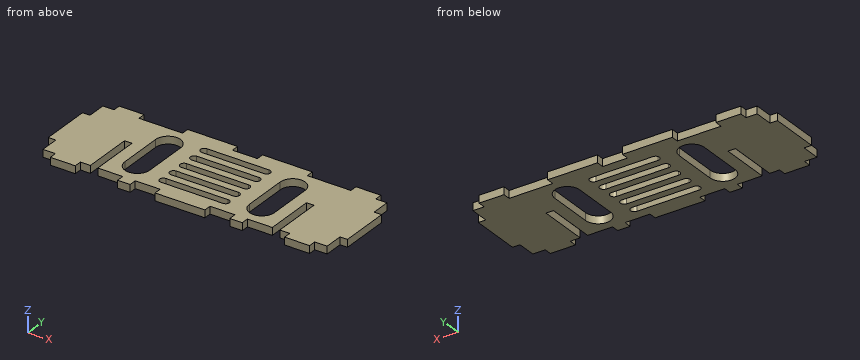
Autodesk Inventor part; units mm, degrees
ref_plane "YZ Plane" through (0, 0, 0) normal (1, 0, 0) x (0, 1, 0)
ref_plane "XZ Plane" through (0, 0, 0) normal (0, 1, 0) x (-1, 0, 0)
ref_plane "XY Plane" through (0, 0, 0) normal (0, 0, 1) x (1, 0, 0)
sketch "Sketch1" plane through (0, 0, 0) normal (0, 0, 1) x (1, 0, 0)
  line L0 (57, -17.5) -> (-57, -17.5)
  line L1 (-57, -17.5) -> (-57, 17.5)
  line L2 (-57, 17.5) -> (57, 17.5)
  line L3 (57, 17.5) -> (57, -17.5)
  line L4 (57, -17.5) -> (-57, 17.5) construction
  line L5 (-57, -17.5) -> (57, 17.5) construction
  point P0 (0, 0)
  dimension "d0" = 114
  dimension "d1" = 35
extrude "Extrusion1" add sketch "Sketch1" along normal blind 3
sketch "Sketch2" plane through (0, 0, 3) normal (0, 0, 1) x (1, 0, 0)
  line L0 (-57, -17.5) -> (57, -17.5)
  line L1 (10, -17.5) -> (-10, -17.5)
  line L2 (-10, -17.5) -> (-10, -20.5)
  line L3 (-10, -20.5) -> (10, -20.5)
  line L4 (10, -20.5) -> (10, -17.5)
  line L5 (-20, -17.5) -> (-25, -17.5)
  line L6 (-25, -17.5) -> (-25, -20.5)
  line L7 (-25, -20.5) -> (-20, -20.5)
  line L8 (-20, -20.5) -> (-20, -17.5)
  line L9 (20, -17.5) -> (25, -17.5)
  line L10 (25, -17.5) -> (25, -20.5)
  line L11 (25, -20.5) -> (20, -20.5)
  line L12 (20, -20.5) -> (20, -17.5)
  point P0 (0, 0)
  point P1 (0, -20.5)
  dimension "d4" = 20
  dimension "d5" = 3
  dimension "d6" = 5
  dimension "d7" = 3
  dimension "d8" = 10
  dimension "d9" = 5
  dimension "d10" = 3
  dimension "d11" = 10
extrude "Extrusion2" add sketch "Sketch2" against normal blind 3
sketch "Sketch3" plane through (0, 0, 0) normal (0, 0, -1) x (-1, 0, 0)
  line L0 (57, -17.5) -> (25, -17.5)
  line L1 (38, -17.5) -> (35, -17.5)
  line L2 (35, -17.5) -> (35, 2.5)
  line L3 (35, 2.5) -> (38, 2.5)
  line L4 (38, 2.5) -> (38, -17.5)
  line L5 (-57, 17.5) -> (57, 17.5)
  point P0 (0, 0)
  dimension "d14" = 3
  dimension "d15" = 15
  dimension "d16" = 35
extrude "Extrusion3" cut sketch "Sketch3" against normal blind 3
sketch "Sketch4" plane through (0, 0, 0) normal (0, 0, -1) x (-1, 0, 0)
  line L0 (38, -17.5) -> (57, -17.5)
  line L1 (42, -17.5) -> (52, -17.5)
  line L2 (52, -17.5) -> (52, -20.5)
  line L3 (52, -20.5) -> (42, -20.5)
  line L4 (42, -20.5) -> (42, -17.5)
  line L5 (25, -20.5) -> (25, -17.5)
  point P0 (0, 0)
  dimension "d19" = 10
  dimension "d20" = 3
  dimension "d21" = 17
extrude "Extrusion4" add sketch "Sketch4" against normal blind 3
sketch "Sketch5" plane through (0, 0, 0) normal (0, 0, -1) x (-1, 0, 0)
  line L0 (57, 17.5) -> (57, -17.5)
  line L1 (57, -10) -> (60, -10)
  line L2 (60, -10) -> (60, 10)
  line L3 (60, 10) -> (57, 10)
  line L4 (57, 10) -> (57, -10)
  line L5 (52, -17.5) -> (57, -17.5)
  point P0 (0, 0)
  dimension "d24" = 3
  dimension "d25" = 20
  dimension "d26" = 7.5
extrude "Extrusion5" add sketch "Sketch5" against normal blind 3
mirror "Mirror1" about plane through (0, 0, 0) normal (1, 0, 0) of "Extrusion5", "Extrusion4", "Extrusion3"
sketch "Sketch6" plane through (0, 0, 3) normal (0, 0, 1) x (1, 0, 0)
  line L0 (-57, 17.5) -> (57, 17.5)
  line L1 (52.5, 17.5) -> (42.5, 17.5)
  line L2 (42.5, 17.5) -> (42.5, 20.5)
  line L3 (42.5, 20.5) -> (52.5, 20.5)
  line L4 (52.5, 20.5) -> (52.5, 17.5)
  line L5 (25, 17.5) -> (5, 17.5)
  line L6 (5, 17.5) -> (5, 20.5)
  line L7 (5, 20.5) -> (25, 20.5)
  line L8 (25, 20.5) -> (25, 17.5)
  point P0 (0, 0)
  dimension "d29" = 10
  dimension "d30" = 3
  dimension "d31" = 20
  dimension "d32" = 3
  dimension "d33" = 17.5
  dimension "d34" = 5
extrude "Extrusion6" add sketch "Sketch6" against normal blind 3
sketch "Sketch7" plane through (0, 0, 3) normal (0, 0, 1) x (1, 0, 0)
  line L0 (25, 9) -> (25, -9) construction
  line L1 (20, 9) -> (20, -9)
  line L2 (30, -9) -> (30, 9)
  arc A0 (30, 9) -> (20, 9) centre (25, 9) ccw
  arc A1 (20, -9) -> (30, -9) centre (25, -9) ccw
  point P0 (0, 0)
  point P1 (25, 0)
  dimension "d37" = 18
  dimension "d38" = 10
  dimension "d39" = 25
extrude "Extrusion7" cut sketch "Sketch7" against normal blind 3
sketch "Sketch8" plane through (0, 0, 3) normal (0, 0, 1) x (1, 0, 0)
  line L0 (12.5, 12) -> (-12.5, 12) construction
  line L1 (12.5, 13.5) -> (-12.5, 13.5)
  line L2 (-12.5, 10.5) -> (12.5, 10.5)
  arc A0 (12.5, 10.5) -> (12.5, 13.5) centre (12.5, 12) ccw
  arc A1 (-12.5, 13.5) -> (-12.5, 10.5) centre (-12.5, 12) ccw
  line L3 (-12.5, 6) -> (12.5, 6) construction
  line L4 (-12.5, 4.5) -> (12.5, 4.5)
  line L5 (12.5, 7.5) -> (-12.5, 7.5)
  arc A2 (-12.5, 7.5) -> (-12.5, 4.5) centre (-12.5, 6) ccw
  arc A3 (12.5, 4.5) -> (12.5, 7.5) centre (12.5, 6) ccw
  line L6 (-12.5, -6) -> (12.5, -6) construction
  line L7 (-12.5, -7.5) -> (12.5, -7.5)
  line L8 (12.5, -4.5) -> (-12.5, -4.5)
  arc A4 (-12.5, -4.5) -> (-12.5, -7.5) centre (-12.5, -6) ccw
  arc A5 (12.5, -7.5) -> (12.5, -4.5) centre (12.5, -6) ccw
  line L9 (-12.5, -12) -> (12.5, -12) construction
  line L10 (-12.5, -13.5) -> (12.5, -13.5)
  line L11 (12.5, -10.5) -> (-12.5, -10.5)
  arc A6 (-12.5, -10.5) -> (-12.5, -13.5) centre (-12.5, -12) ccw
  arc A7 (12.5, -13.5) -> (12.5, -10.5) centre (12.5, -12) ccw
  line L12 (-12.5, 0) -> (12.5, 0) construction
  line L13 (-12.5, -1.5) -> (12.5, -1.5)
  line L14 (12.5, 1.5) -> (-12.5, 1.5)
  arc A8 (-12.5, 1.5) -> (-12.5, -1.5) centre (-12.5, 0) ccw
  arc A9 (12.5, -1.5) -> (12.5, 1.5) centre (12.5, 0) ccw
  point P0 (0, 0)
  point P1 (0, 12)
  point P2 (0, 6)
  point P3 (0, -6)
  point P4 (0, -12)
  point P5 (0, 0)
  dimension "d42" = 3
  dimension "d43" = 12
  dimension "d44" = 3
  dimension "d45" = 3
  dimension "d46" = 3
  dimension "d47" = 12
  dimension "d48" = 6
  dimension "d49" = 6
  dimension "d50" = 3
  dimension "d51" = 25
extrude "Extrusion8" cut sketch "Sketch8" against normal blind 3
mirror "Mirror2" about plane through (0, 0, 0) normal (1, 0, 0) of "Extrusion6", "Extrusion7"
equation "\"d11\" = d8"
properties part number "Lower bottom"
Geometry check sheet. Reference: the model listing, model coordinates, mm. Round coordinates to 2 decimals unless told otherwise and drop trailing zeros. Order: outer loops, then holes, each group sorted by start corner. A loop starts at its lowest first (then second) coordinate and runs counter-clockwise, first axis right, second up. Notation, with made-up numbers: (79.25, -10.5) -> (125.25, -10.5) arc R24 cw to (125.25, 20.5) -> close; hole circle Ø1 at (69, 37). An arc over 180 degrees is marked (long way). Use one line per item in the form item = value.
1. Go/stop test with flat-tipped pins: pin 1 (1.5 mm diameter, centred on x = -58.5, z = 1, fed in from +Y); pin 2 (1 mm diameter, centred on x = -18, z = 1.5, fed in from -Y). Record where each tip stops, or that it passes through.
Working result:
pin_1 = 10
pin_2 = -17.5
2. Cross-section at B-B, the plane y = -12. Enter the section's corners in (x, z), plus the area to 3 significant figures.
Working result:
outline = (-57, 0) -> (-38, 0) -> (-38, 3) -> (-57, 3) -> close; (-35, 0) -> (-29, 0) -> (-29, 3) -> (-35, 3) -> close; (-21, 0) -> (-14, 0) -> (-14, 3) -> (-21, 3) -> close; (14, 0) -> (21, 0) -> (21, 3) -> (14, 3) -> close; (29, 0) -> (35, 0) -> (35, 3) -> (29, 3) -> close; (38, 0) -> (57, 0) -> (57, 3) -> (38, 3) -> close
area = 192 mm^2
3. Cross-section at A-A, the plane y = 12. Enter the section's corners in (x, z).
Working result:
outline = (-57, 0) -> (-29, 0) -> (-29, 3) -> (-57, 3) -> close; (-21, 0) -> (-14, 0) -> (-14, 3) -> (-21, 3) -> close; (14, 0) -> (21, 0) -> (21, 3) -> (14, 3) -> close; (29, 0) -> (57, 0) -> (57, 3) -> (29, 3) -> close
4. Scan lines: line 1 along Y through (x, z) = (2, 0.65); line 2 along X through (y, z) = (6, 0.6); line 3 along X through (y, z) = (-4, 1). Record each from-to range of solid material in increasing order. Write a range as from..to.
Working result:
line_1 = -20.5..-13.5, -10.5..-7.5, -4.5..-1.5, 1.5..4.5, 7.5..10.5, 13.5..17.5
line_2 = -60..-30, -20..-14, 14..20, 30..60
line_3 = -60..-38, -35..-30, -20..20, 30..35, 38..60
5. Cross-section at D-D, the plane z = 0.5. Count the separate pieces of the cut face and the enclosed holes in it, plus the area to 3 significant figures.
Working result:
separate_pieces = 1
enclosed_holes = 7
area = 3,390 mm^2
6. Cross-section at C-C, the plane x = -36.5. Enter the section's corners in (y, z), plus the area to 3 significant figures.
Working result:
outline = (2.5, 0) -> (17.5, 0) -> (17.5, 3) -> (2.5, 3) -> close
area = 45.0 mm^2
